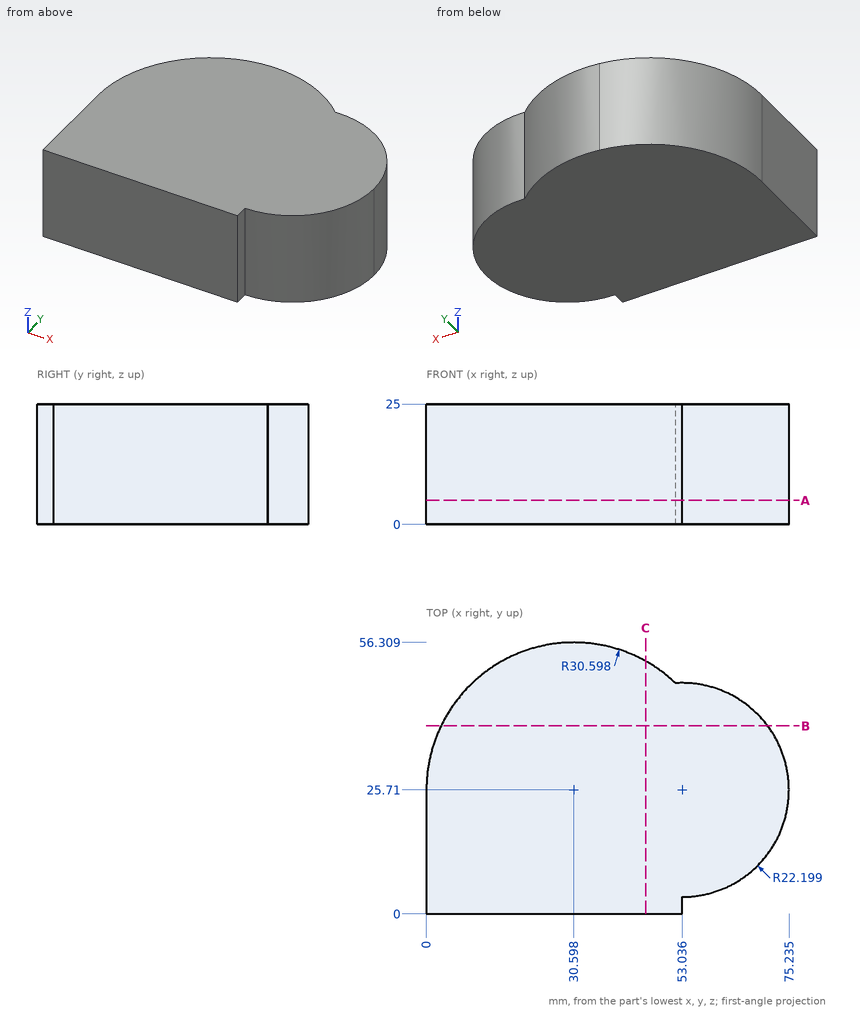
For this review, use the dimensioned drawing (mm, ordinates from the lowest corner) and the shaded views. Round coordinates to 2 decimals unless told otherwise and drop trailing zeros. Order: outer loops, then holes, each group sorted by start corner. A loop starts at its lowest first (then second) coordinate and runs counter-clockwise, first axis right, second up. Notation, with made-up numbers: M 52.25,65.25 L 69.25,65.25 A36 ccw 69.25,104.25 Z; hole C 48.5,-40 d4. An arc over 180 degrees is marked long. Use a Markdown table: item, result.
1) Wall thickness on line 1 along X through (y, z) = (29, 8); line 2 along X through (y, z) = (10, 21.5); line 3 along Y through (x, z) = (66, 14.75): over which ranges is each line inside the solid? List them lowest first. Write a range as [from, to].
Report:
| item | result |
|---|---|
| line 1 | [0.18, 74.99] |
| line 2 | [0, 68.72] |
| line 3 | [7.69, 43.73] |
2) Insertion check: pin 1 (3 mm diameter, centred on y = 1, z = 17, fed in from +X); pin 2 (1 mm diameter, centred on y = 10, z = 19, fed in from +X) (1 decimal); pin 3 (1.5 mm diameter, centred on x = 8.5, y = 8, fed in from -Z); pin 4 (1 mm diameter, centred on x = 27.5, z = 6.5, fed in from +Y). Each pin has a flat end and moves straight along its axis. Give the tip position at first contact, or say it passes through.
Report:
| item | result |
|---|---|
| pin 1 | x = 53.04 |
| pin 2 | x = 69.2 |
| pin 3 | z = 0 |
| pin 4 | y = 56.2 |
3) Consider section C-C (x = 45.5). Write out the cut boundary in (y, z) (1 decimal), then the cut area to 3 significant figures.
Report:
| item | result |
|---|---|
| outline | M 0,0 L 52.4,0 L 52.4,25 L 0,25 Z |
| area | 1,310 mm^2 |
4) Consider section B-B (y = 39). Write out the cut boundary in (x, z).
Report:
| item | result |
|---|---|
| outline | M 3.04,0 L 70.82,0 L 70.82,25 L 3.04,25 Z |
5) Consider section A-A (z = 5). Write out the cut boundary in (x, y) (1 decimal).
Report:
| item | result |
|---|---|
| outline | M 0,0 L 53,0 L 53,3.5 A22.2 ccw long 51.7,47.9 A30.6 ccw 0,25.7 Z |
